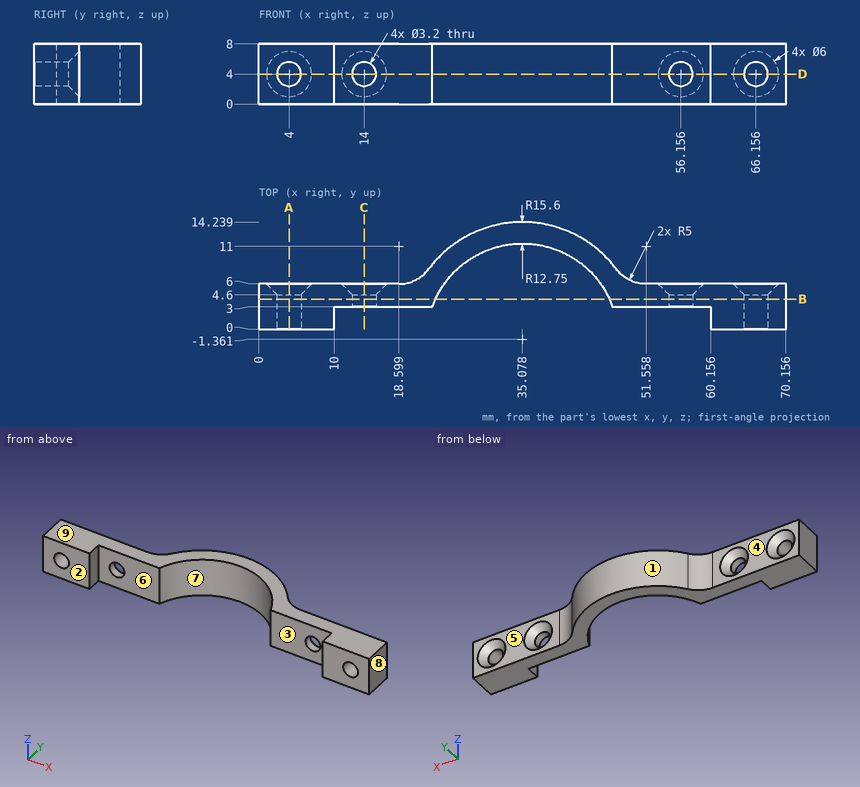
For this review, use the dimensioned drawing (mm, ordinates from the lowest corner) and the shaded views. A direction names the side the tool comes from. Give positions to 0.01 mm unless a question says otherwise; leave off trailing zeros. Write each loop counter-clockwise with the first axis right and the second up, starting at its lowest first coordinate (ties: lowest second). Pieces come first, ordered by that corner, then holes. Notation, with made-up numbers: M 87.5,87.5 L 124.5,87.5 A15 ccw 124.5,105.5 Z; hole C 6,41 d11. An arc over 180 degrees is marked long. Answer as a JSON object with one key per item and string values. Group by question number.
Item 1: Consider section C-C on x = 14. Write out the cut boundary in (y, z).
Item 2: Consider section D-D on z = 4. Count the separate pieces of the cut face and the enclosed holes in it, plus the area to 3 significant figures.
Item 3: Tool access review of the marked faces 1, 2, 3, 4 and 5: name each direction out of +Z, -Z, +X, -X, +Y, -Y from which nothing blocks a thin tool from reaching the whole face with its end or side.
Item 4: Draft analysis for pull direction X (two halves, no side actions). For the marked faces 6, 7, 8 and 9, state which applies: +X half, -X half, draft (parallel to the pull), parting line (faces both ways), or undercut.
Item 5: Consider section A-A on x = 4. Write out the cut boundary in (y, z).
Item 6: Consider section B-B on y = 4. Write out the cut boundary in (x, z), plus the area to 3 significant figures.
Item 7: For pin 1 Ø4 at (x, z) = (4, 4) entering from +Y; pin 2 Ø2.5 at (x, z) = (9.5, 2.5) entering from +Y; pin 3 Ø3 at (y, z) = (11.5, 7) entering from +X, all flat-tipped, find the tip position at first contact; note any pin that passes through.
Item 8: For probe 1 along X at (y, z) = (1, 4); probe 2 along Z at (x, y) = (14, 3.6); probe 3 along X at (y, z) = (4.75, 4.5) (1 decimal), list the stretches that pass through material, from the lowest coordinate up. Write a range as [from, to].
Check result:
{
 "1": {"outline": "M 3,0 L 6,0 L 6,1 L 4.6,2.4 L 3,2.4 Z; M 3,5.6 L 4.6,5.6 L 6,7 L 6,8 L 3,8 Z"},
 "2": {"separate pieces": "5", "enclosed holes": "0", "area": "222 mm^2"},
 "3": {"face 1": "+Z, -Z, +Y", "face 2": "+Z, -Z, +X, -X, -Y", "face 3": "+Z, -Z, -Y", "face 4": "+Z, -Z, -X, +Y", "face 5": "+Z, -Z, +X, +Y"},
 "4": {"face 6": "undercut", "face 7": "undercut", "face 8": "+X half", "face 9": "draft"},
 "5": {"outline": "M 0,0 L 6,0 L 6,1 L 4.6,2.4 L 0,2.4 Z; M 0,5.6 L 4.6,5.6 L 6,7 L 6,8 L 0,8 Z"},
 "6": {"outline": "M 0,0 L 23.51,0 L 23.51,8 L 0,8 Z; M 46.65,0 L 70.16,0 L 70.16,8 L 46.65,8 Z; hole C 4,4 d3.2; hole C 14,4 d3.2; hole C 56.16,4 d3.2; hole C 66.16,4 d3.2", "area": "344 mm^2"},
 "7": {"pin 1": "stops at y = 5", "pin 2": "stops at y = 6", "pin 3": "stops at x = 45.77"},
 "8": {"probe 1": "x = [0, 2.4], [5.6, 10], [60.16, 64.56], [67.76, 70.16]", "probe 2": "z = [0, 2.4], [5.6, 8]", "probe 3": "x = [0, 2.3], [5.7, 12.3], [15.7, 23.9], [46.3, 54.5], [57.8, 64.5], [67.8, 70.2]"}
}
